```python
from build123d import *

# Parameters (mm, degrees)
F1_DEPTH = 5
F2_DEPTH = 5
F3_DEPTH = 100
F4_DEPTH = 100
F5_R     = 4.25
F6_DEPTH = 10
F7_R     = 2


with BuildPart() as f1:
    # F0 (on Front) → F1 (new body)
    with BuildSketch(Plane.XZ):
        Polygon((-33.825879693, 2.8445311606), (-33.825879693, -67.1554688394), (36.174120307, 2.8445311606), align=None)
    extrude(amount=F1_DEPTH)

    # F0 (on Front) → F2 (join)
    with BuildSketch(Plane.XZ):
        Polygon((-33.825879693, 2.8445311606), (-33.825879693, -67.1554688394), (36.174120307, 2.8445311606), align=None)
    extrude(amount=-F2_DEPTH)

    # F0 (on Front) → F3 (join)
    with BuildSketch(Plane.XZ):
        Polygon((-43.825879693, 89.6445311606), (-43.825879693, -110.3554688394), (-33.825879693, -110.3554688394), (-33.825879693, -67.1554688394), (-33.825879693, 2.8445311606), (36.174120307, 2.8445311606), (66.174120307, 2.8445311606), (66.174120307, 12.8445311606), (-33.825879693, 12.8445311606), (-33.825879693, 89.6445311606), align=None)
    extrude(amount=F3_DEPTH)

    # F4 (add): a face of the model
    f4_faces = [f1.faces().sort_by_distance(p)[0] for p in [
        (-41.5433372509, 0, -10.3554688394),
    ]]
    extrude(f4_faces, amount=F4_DEPTH)

    # F5 (on face) → F6 (cut)
    with BuildSketch(Plane.YZ.offset(-33.825879693)):
        with Locations((-85, -95.3554688394)):
            Circle(F5_R)
        with Locations((85, -95.3554688394)):
            Circle(F5_R)
        with Locations((85, 74.6445311606)):
            Circle(F5_R)
        with Locations((-85, 74.6445311606)):
            Circle(F5_R)
    extrude(amount=-F6_DEPTH, mode=Mode.SUBTRACT)

    # F7
    f7_edges = [f1.edges().sort_by_distance(p)[0] for p in [
        (-33.82588, -52.5, 2.844531),
        (-33.82588, 52.5, 2.844531),
        (1.17412, 5, 2.844531),
        (-33.82588, 5, -32.155469),
        (1.17412, -5, 2.844531),
        (-33.82588, -5, -32.155469),
        (-33.82588, 0, 12.844531),
    ]]
    fillet(f7_edges, radius=F7_R)


solid = f1.part
```
Work out the finished part from the listing and answer in its coordinate system (mm). A direction names the side the tool comes from. Round coordinates to 2 decimals unless told otherwise and drop trailing zeros. Write each loop counter-clockwise with the first axis right and the second up, starting at its lowest first coordinate (ties: lowest second). Pieces come first, ordered by that corner, then holes. Notation, with made-up numbers: (29, -39.5) - (85, -39.5) arc R26 cw to (85, -15.5) - close; hole circle Ø4 at (-37, 40). An arc over 180 degrees is marked (long way). Return JSON: item names as keys, results as strings. Group by question number.
Q1. The part is cut by section A-A on y = 85. Write down the section's boundary in (x, z).
Q2. The mould has two halves that part along Y. Classify faces 1 (the flat face through (-18, 100, 5)), 2 (the flat face through (-39, -1, 89.645)), 3 (the flat face through (-18, -100, 5)), 4 (the cylindrical face through (-38.76, -85.55, -91.14)): released by +Y, released by -Y, zero draft, split by the parting line, or undercut.
Q3. Each of these flat-tipped pins is pushed along its axis until it touches: pin 1 Ø1 at (y, z) = (-27, -41) entering from +X; pin 2 Ø6 at (x, y) = (6.5, 65) entering from +Z; pin 3 Ø5 at (y, z) = (85, 74.64) entering from +X; pin 4 Ø12 at (x, y) = (33.5, -58.5) entering from -Z. Where does it stop, or does it pass through?
Q4. Find the intervals of material crossed by L1, parallel to Z at x = -41.5, y = -85; L2, parallel to X at y = -65, z = 58.5; L3, parallel to Y at x = -11, z = -22, in increasing order.
Q5. For faces 5 (the flat face through (-7, -5, -24)), 6 (the flat face through (-33.826, -1, -68)), 7 (the flat face through (-7, 5, -24)), 8 (the flat face through (-33.826, -1, 52)), 9 (the flat face through (-43.826, -1, -9)), determine the directions among +Z, -Z, +X, -X, +Y, -Y from which every point of the face is accessible in a straight line to the end or side of a thin tool.
Q6. The part is cut by section C-C on x = 24. Write down the section's boundary in (y, z), then the cut area to 3 significant figures.
Q7. The part is cut by section D-D on z = 59. Write down the section's boundary in (x, y), then the cut area to 3 significant figures.
Q8. The part is cut by section B-B on y = -64.5. Write down the section's boundary in (x, z).
Solved:
{
 "1": {"outline": "(-43.83, -110.36) - (-33.83, -110.36) - (-33.83, -99.61) - (-43.83, -99.61) - close; (-43.83, -91.11) - (-33.83, -91.11) - (-33.83, 0.84) arc R2 cw to (-31.83, 2.84) - (66.17, 2.84) - (66.17, 12.84) - (-31.83, 12.84) arc R2 cw to (-33.83, 14.84) - (-33.83, 70.39) - (-43.83, 70.39) - close; (-43.83, 78.89) - (-33.83, 78.89) - (-33.83, 89.64) - (-43.83, 89.64) - close"},
 "2": {"face 1": "released by +Y", "face 2": "zero draft", "face 3": "released by -Y", "face 4": "undercut"},
 "3": {"pin 1": "x = -33.83", "pin 2": "z = 12.84", "pin 3": "through", "pin 4": "z = 2.84"},
 "4": {"L1": "-110.36 to -99.61, -91.11 to 70.39, 78.89 to 89.64", "L2": "-43.83 to -33.83", "L3": "-5 to 5"},
 "5": {"face 5": "-Z, +X, -Y", "face 6": "-Z, +X", "face 7": "-Z, +X, +Y", "face 8": "+Z, +X, +Y, -Y", "face 9": "+Z, -Z, -X, +Y, -Y"},
 "6": {"outline": "(-100, 2.84) - (-7, 2.84) arc R2 cw to (-5, 0.84) - (-5, -9.33) - (5, -9.33) - (5, 0.84) arc R2 cw to (7, 2.84) - (100, 2.84) - (100, 12.84) - (-100, 12.84) - close", "area": "2,120 mm²"},
 "7": {"outline": "(-43.83, -100) - (-33.83, -100) - (-33.83, 100) - (-43.83, 100) - close", "area": "2,000 mm²"},
 "8": {"outline": "(-43.83, -110.36) - (-33.83, -110.36) - (-33.83, 0.84) arc R2 cw to (-31.83, 2.84) - (66.17, 2.84) - (66.17, 12.84) - (-31.83, 12.84) arc R2 cw to (-33.83, 14.84) - (-33.83, 89.64) - (-43.83, 89.64) - close"}
}
